The model under review builds one solid part; all positions refer to its coordinate system, in mm. A direction names the side the tool comes from. Coordinates: 2 decimals unless noted, no trailing zeros. Loops run counter-clockwise (first coordinate to the right, second up) from the corner with the lowest first, then second, coordinate; pieces in that order, holes last. Notation, with made-up numbers: (77, 75) -> (133, 75) arc R31 ccw to (133, 103) -> close; hole circle Ø2 at (-39.5, 63.5). An arc over 180 degrees is marked (long way). One line per question, with ' | ' between items. Start each with the question number.
Autodesk Inventor part; units mm, degrees
ref_plane "YZ Plane" through (0, 0, 0) normal (1, 0, 0) x (0, 1, 0)
ref_plane "XZ Plane" through (0, 0, 0) normal (0, 1, 0) x (-1, 0, 0)
ref_plane "XY Plane" through (0, 0, 0) normal (0, 0, 1) x (1, 0, 0)
sketch "Szkic1" plane through (0, 0, 0) normal (0, 0, 1) x (1, 0, 0)
  circle A0 centre (0, 0) radius 14
  dimension "d0" = 28
extrude "Wyciągnięcie proste1" add sketch "Szkic1" along normal blind 27.5
sketch "Szkic2" plane through (0, 0, 0) normal (0, 0, -1) x (-1, 0, 0)
  circle A0 centre (0, 0) radius 8
  circle A1 centre (0, 0) radius 14
  dimension "d3" = 16
extrude "Wyciągnięcie proste2" cut sketch "Szkic2" against normal blind 14
sketch "Szkic3" plane through (0, 0, 0) normal (0, 0, -1) x (-1, 0, 0)
  circle A0 centre (0, 0) radius 8
  circle A1 centre (0, 0) radius 5
  dimension "d6" = 10
extrude "Wyciągnięcie proste3" cut sketch "Szkic3" against normal up to next contours A1
sketch "Szkic4" plane through (0, 0, 27.5) normal (0, 0, 1) x (1, 0, 0)
  line L0 (0, 0) -> (0, 9.5)
  circle A0 centre (0, 9.5) radius 2
  circle A1 centre (0, 0) radius 14
  circle A2 centre (8.2272, 4.75) radius 2
  circle A3 centre (8.2272, -4.75) radius 2
  circle A4 centre (0, -9.5) radius 2
  circle A5 centre (-8.2272, -4.75) radius 2
  circle A6 centre (-8.2272, 4.75) radius 2
  dimension "d9" = 9.5
  dimension "d10" = 4
  dimension "d13" = 360
extrude "Wyciągnięcie proste4" cut sketch "Szkic4" against normal blind 12 contours A0 | A2 | A3 | A4 | A5 | A6
thread "Gwint1"
thread "Gwint2"
thread "Gwint3"
thread "Gwint4"
thread "Gwint5"
thread "Gwint6"
properties part number "Tuleja zaciskowo rozprężna RCK BK 80 10x16 Clampex"
1) Consider section B-B, the plane z = 19. Write out the cut boundary in (x, y), plus the area to 3 significant figures.
2) Mouldability with a two-part tool opening along Y and no side actions: class faces 1 (the face through (6.64, -5.97, 21.58)), 2 (the face through (-6.38, -5.52, 21.58)), 3 (the face through (1.73, -7.81, 6.9)), 4 (the face through (-6, -6, 14)) as +Y half, -Y half, draft (parallel to the pull), parting line (faces both ways), or undercut.
3) Consider section D-D, the plane x = 3.75. Write out the cut boundary in (y, z).
4) Consider section C-C, the plane x = 0. Write out the cut boundary in (y, z).
5) Machinability: for faces 5 (the face through (12.932, 5.362, 20.656)), 6 (the face through (-8, -5, 15.5)), which of the approach directions +Z, -Z, +X, -X, +Y, -Y give a long, thin tool a straight path to every point of the face, cutting with its end or side? Answer none if there is none.
6) Consider section A-A, the plane y = 0. Write out the cut boundary in (x, z).
7) Wall thickness on L1, parallel to Y at x = 0, z = 20.25; L2, parallel to Y at x = -1.75, z = 16; L3, parallel to Y at x = -6.5, z = 20.25: over which ranges is each line inside the solid? List them lowest first.
8) Insertion check: pin 1 Ø3 at (x, y) = (-8.23, -4.75) entering from +Z; pin 2 Ø3 at (x, y) = (-7.5, -5.5) entering from +Z; pin 3 Ø3 at (x, z) = (-2.5, 23.5) entering from +Y; pin 4 Ø2.5 at (x, y) = (0, 9.5) entering from -Z. Each pin has a flat end and moves straight along its axis. Give the tip position at first contact, or say it passes through.
Filled sheet:
1) outline: circle Ø28 at (0, 0); hole circle Ø4 at (-8.23, -4.75); hole circle Ø4 at (-8.23, 4.75); hole circle Ø10 at (0, 0); hole circle Ø4 at (0, -9.5); hole circle Ø4 at (0, 9.5); hole circle Ø4 at (8.23, -4.75); hole circle Ø4 at (8.23, 4.75) | area: 462 mm^2
2) face 1: undercut | face 2: undercut | face 3: parting line | face 4: draft
3) outline: (-13.49, 14) -> (-7.07, 14) -> (-7.07, 0) -> (-3.31, 0) -> (-3.31, 27.5) -> (-13.49, 27.5) -> close; (3.31, 0) -> (7.07, 0) -> (7.07, 14) -> (13.49, 14) -> (13.49, 27.5) -> (3.31, 27.5) -> close
4) outline: (-14, 14) -> (-8, 14) -> (-8, 0) -> (-5, 0) -> (-5, 27.5) -> (-7.5, 27.5) -> (-7.5, 15.5) -> (-11.5, 15.5) -> (-11.5, 27.5) -> (-14, 27.5) -> close; (5, 0) -> (8, 0) -> (8, 14) -> (14, 14) -> (14, 27.5) -> (11.5, 27.5) -> (11.5, 15.5) -> (7.5, 15.5) -> (7.5, 27.5) -> (5, 27.5) -> close
5) face 5: +Z, -Z | face 6: +Z
6) outline: (-14, 14) -> (-8, 14) -> (-8, 0) -> (-5, 0) -> (-5, 27.5) -> (-14, 27.5) -> close; (5, 0) -> (8, 0) -> (8, 14) -> (14, 14) -> (14, 27.5) -> (5, 27.5) -> close
7) L1: -14 to -11.5, -7.5 to -5, 5 to 7.5, 11.5 to 14 | L2: -13.89 to -10.47, -8.53 to -4.68, 4.68 to 8.53, 10.47 to 13.89 | L3: -12.4 to -5.76, -3.74 to 3.74, 5.76 to 12.4
8) pin 1: z = 15.5 | pin 2: z = 27.5 | pin 3: y = 13.96 | pin 4: z = 14
